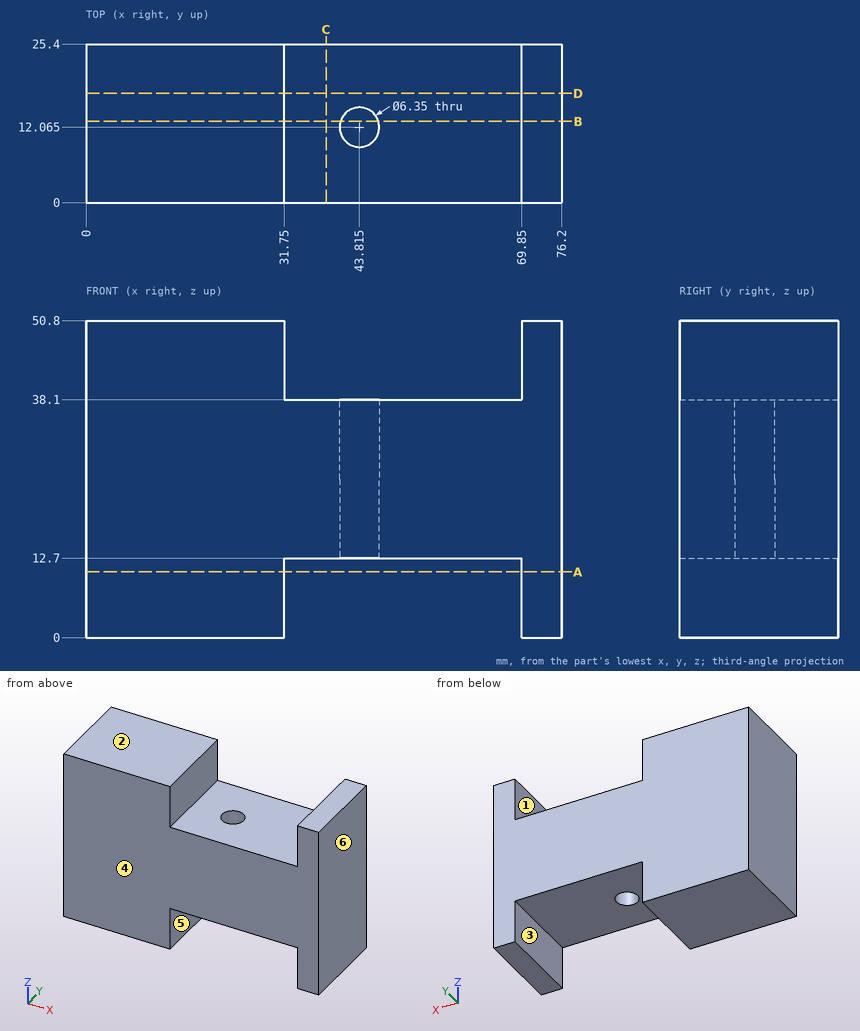
For this review, use the dimensioned drawing (mm, ordinates from the lowest corner) and the shaded views. A direction names the side the tool comes from. Give positions to 0.01 mm unless a question says otherwise; leave off trailing zeros. Write each loop counter-clockwise with the first axis right and the second up, starting at its lowest first coordinate (ties: lowest second). Pieces come first, ordered by that corner, then holes.
(1) Consider section B-B, the plane y = 13. Give the boundary of the cut face in (x, z).
(2) Tool access review of the marked faces 1, 2 and 3: name each direction out of +Z, -Z, +X, -X, +Y, -Y from which nothing blocks a thin tool from reaching the whole face with its end or side.
(3) Consider section A-A, the plane z = 10.5. Give the boundary of the cut face in (x, y), and give its area (3 significant figures).
(4) Consider section D-D, the plane y = 17.5. Give the boundary of the cut face in (x, z).
(5) For P1, Ø5, axis at x = 67, y = 12.5, coming from the +Z side; P2, Ø5, axis at x = 43.815, y = 12.065, coming from the -Z side; P3, Ø10, axis at x = 38, y = 12, coming from the -Z side, all flat-tipped, find the tip position at first contact; note any pin that passes through.
(6) To check wall thickness, follow L1, parallel to X at y = 6, z = 38.5; L2, parallel to Z at x = 34, y = 15; L3, parallel to X at y = 10, z = 34. State the ranges of each line that lie inside material, in increasing order.
(7) The part is to be moulded in two halves that separate along X. For the marked faces 4, 5 and 6, say which applies: released by +X, released by -X, zero draft, split by the parting line, or undercut.
(8) Consider section C-C, the plane x = 38.5. Give the boundary of the cut face in (y, z), and give its area (3 significant figures).
Returned:
1. outline: (0, 0) - (31.75, 0) - (31.75, 12.7) - (40.78, 12.7) - (40.78, 38.1) - (31.75, 38.1) - (31.75, 50.8) - (0, 50.8) - close; (46.85, 12.7) - (69.85, 12.7) - (69.85, 0) - (76.2, 0) - (76.2, 50.8) - (69.85, 50.8) - (69.85, 38.1) - (46.85, 38.1) - close
2. face 1: +Z, +Y, -Y
2. face 2: +Z, +X, -X, +Y, -Y
2. face 3: -Z, +Y, -Y
3. outline: (0, 0) - (31.75, 0) - (31.75, 25.4) - (0, 25.4) - close; (69.85, 0) - (76.2, 0) - (76.2, 25.4) - (69.85, 25.4) - close
3. area: 968 mm2
4. outline: (0, 0) - (31.75, 0) - (31.75, 12.7) - (69.85, 12.7) - (69.85, 0) - (76.2, 0) - (76.2, 50.8) - (69.85, 50.8) - (69.85, 38.1) - (31.75, 38.1) - (31.75, 50.8) - (0, 50.8) - close
5. P1: stops at z = 38.1
5. P2: passes through
5. P3: stops at z = 12.7
6. L1: x = 0 to 31.75, 69.85 to 76.2
6. L2: z = 12.7 to 38.1
6. L3: x = 0 to 41.4, 46.23 to 76.2
7. face 4: zero draft
7. face 5: undercut
7. face 6: released by +X
8. outline: (0, 12.7) - (25.4, 12.7) - (25.4, 38.1) - (0, 38.1) - close
8. area: 645 mm2
